Autodesk Inventor part; units mm, degrees
ref_plane "YZ Plane" through (0, 0, 0) normal (1, 0, 0) x (0, 1, 0)
ref_plane "XZ Plane" through (0, 0, 0) normal (0, 1, 0) x (-1, 0, 0)
ref_plane "XY Plane" through (0, 0, 0) normal (0, 0, 1) x (1, 0, 0)
sketch "Sketch4" plane through (0, 0, 0) normal (1, 0, 0) x (0, 1, 0)
  ellipse E0 centre (0, 0) end of major axis (-20, 0) minor radius 10
  dimension "d32" = 20
  dimension "d33" = 10
extrude "Extrusion1" add sketch "Sketch4" along normal blind 280
sketch "Sketch5" plane through (0, 0, 0) normal (-1, 0, 0) x (0, 0, 1)
  ellipse E0 centre (0, 0) end of major axis (0, 40) minor radius 40
  ellipse E1 centre (0, 0) end of major axis (0, -20) minor radius 10
  line L0 (0, 0) -> (0, 40)
  line L1 (0, 0) -> (-20, 34.641)
  line L2 (0, 0) -> (-34.641, 20)
  line L3 (0, 0) -> (-40, 0)
  line L4 (0, 0) -> (-34.641, -20)
  line L5 (0, 0) -> (-20, -34.641)
  line L6 (0, 0) -> (0, -40)
  line L7 (0, 0) -> (20, -34.641)
  line L8 (0, 0) -> (34.641, -20)
  line L9 (0, 0) -> (40, 0)
  line L10 (0, 0) -> (34.641, 20)
  line L11 (0, 0) -> (20, 34.641)
  line L12 (0, 23.094) -> (3.6979, 33.254)
  line L13 (2.2062, 35.3845) -> (0, 35.3845)
  arc A0 (3.6979, 33.254) -> (2.2062, 35.3845) centre (2.2062, 33.797) ccw
  line L14 (0, 23.094) -> (-3.6979, 33.254)
  line L15 (-2.2062, 35.3845) -> (0, 35.3845)
  arc A1 (-2.2062, 35.3845) -> (-3.6979, 33.254) centre (-2.2062, 33.797) ccw
  line L16 (-15.7816, 31.7469) -> (-17.6922, 30.6438)
  line L17 (-19.6028, 29.5408) -> (-17.6922, 30.6438)
  arc A2 (-19.6028, 29.5408) -> (-19.8295, 26.9498) centre (-18.8091, 28.1659) ccw
  line L18 (-11.547, 20) -> (-19.8295, 26.9498)
  line L19 (-11.547, 20) -> (-13.4245, 30.6478)
  arc A3 (-13.4245, 30.6478) -> (-15.7816, 31.7469) centre (-14.9879, 30.3721) ccw
  line L20 (-29.5408, 19.6028) -> (-30.6438, 17.6922)
  line L21 (-31.7469, 15.7816) -> (-30.6438, 17.6922)
  arc A4 (-31.7469, 15.7816) -> (-30.6478, 13.4245) centre (-30.3721, 14.9879) ccw
  line L22 (-20, 11.547) -> (-30.6478, 13.4245)
  line L23 (-20, 11.547) -> (-26.9498, 19.8295)
  arc A5 (-26.9498, 19.8295) -> (-29.5408, 19.6028) centre (-28.1659, 18.8091) ccw
  line L24 (-35.3845, 2.2062) -> (-35.3845, 0)
  line L25 (-35.3845, -2.2062) -> (-35.3845, 0)
  arc A6 (-35.3845, -2.2062) -> (-33.254, -3.6979) centre (-33.797, -2.2062) ccw
  line L26 (-23.094, 0) -> (-33.254, -3.6979)
  line L27 (-23.094, 0) -> (-33.254, 3.6979)
  arc A7 (-33.254, 3.6979) -> (-35.3845, 2.2062) centre (-33.797, 2.2062) ccw
  line L28 (-31.7469, -15.7816) -> (-30.6438, -17.6922)
  line L29 (-29.5408, -19.6028) -> (-30.6438, -17.6922)
  arc A8 (-29.5408, -19.6028) -> (-26.9498, -19.8295) centre (-28.1659, -18.8091) ccw
  line L30 (-20, -11.547) -> (-26.9498, -19.8295)
  line L31 (-20, -11.547) -> (-30.6478, -13.4245)
  arc A9 (-30.6478, -13.4245) -> (-31.7469, -15.7816) centre (-30.3721, -14.9879) ccw
  line L32 (-19.6028, -29.5408) -> (-17.6922, -30.6438)
  line L33 (-15.7816, -31.7469) -> (-17.6922, -30.6438)
  arc A10 (-15.7816, -31.7469) -> (-13.4245, -30.6478) centre (-14.9879, -30.3721) ccw
  line L34 (-11.547, -20) -> (-13.4245, -30.6478)
  line L35 (-11.547, -20) -> (-19.8295, -26.9498)
  arc A11 (-19.8295, -26.9498) -> (-19.6028, -29.5408) centre (-18.8091, -28.1659) ccw
  line L36 (-2.2062, -35.3845) -> (0, -35.3845)
  line L37 (2.2062, -35.3845) -> (0, -35.3845)
  arc A12 (2.2062, -35.3845) -> (3.6979, -33.254) centre (2.2062, -33.797) ccw
  line L38 (0, -23.094) -> (3.6979, -33.254)
  line L39 (0, -23.094) -> (-3.6979, -33.254)
  arc A13 (-3.6979, -33.254) -> (-2.2062, -35.3845) centre (-2.2062, -33.797) ccw
  line L40 (15.7816, -31.7469) -> (17.6922, -30.6438)
  line L41 (19.6028, -29.5408) -> (17.6922, -30.6438)
  arc A14 (19.6028, -29.5408) -> (19.8295, -26.9498) centre (18.8091, -28.1659) ccw
  line L42 (11.547, -20) -> (19.8295, -26.9498)
  line L43 (11.547, -20) -> (13.4245, -30.6478)
  arc A15 (13.4245, -30.6478) -> (15.7816, -31.7469) centre (14.9879, -30.3721) ccw
  line L44 (29.5408, -19.6028) -> (30.6438, -17.6922)
  line L45 (31.7469, -15.7816) -> (30.6438, -17.6922)
  arc A16 (31.7469, -15.7816) -> (30.6478, -13.4245) centre (30.3721, -14.9879) ccw
  line L46 (20, -11.547) -> (30.6478, -13.4245)
  line L47 (20, -11.547) -> (26.9498, -19.8295)
  arc A17 (26.9498, -19.8295) -> (29.5408, -19.6028) centre (28.1659, -18.8091) ccw
  line L48 (35.3845, -2.2062) -> (35.3845, 0)
  line L49 (35.3845, 2.2062) -> (35.3845, 0)
  arc A18 (35.3845, 2.2062) -> (33.254, 3.6979) centre (33.797, 2.2062) ccw
  line L50 (23.094, 0) -> (33.254, 3.6979)
  line L51 (23.094, 0) -> (33.254, -3.6979)
  arc A19 (33.254, -3.6979) -> (35.3845, -2.2062) centre (33.797, -2.2062) ccw
  line L52 (31.7469, 15.7816) -> (30.6438, 17.6922)
  line L53 (29.5408, 19.6028) -> (30.6438, 17.6922)
  arc A20 (29.5408, 19.6028) -> (26.9498, 19.8295) centre (28.1659, 18.8091) ccw
  line L54 (20, 11.547) -> (26.9498, 19.8295)
  line L55 (20, 11.547) -> (30.6478, 13.4245)
  arc A21 (30.6478, 13.4245) -> (31.7469, 15.7816) centre (30.3721, 14.9879) ccw
  line L56 (19.6028, 29.5408) -> (17.6922, 30.6438)
  line L57 (15.7816, 31.7469) -> (17.6922, 30.6438)
  arc A22 (15.7816, 31.7469) -> (13.4245, 30.6478) centre (14.9879, 30.3721) ccw
  line L58 (11.547, 20) -> (13.4245, 30.6478)
  line L59 (11.547, 20) -> (19.8295, 26.9498)
  arc A23 (19.8295, 26.9498) -> (19.6028, 29.5408) centre (18.8091, 28.1659) ccw
  line L60 (-3.175, 3.5066) -> (3.175, 3.5066)
  line L61 (3.175, 3.5066) -> (3.175, -3.5066)
  line L62 (3.175, -3.5066) -> (-3.175, -3.5066)
  line L63 (-3.175, -3.5066) -> (-3.175, 3.5066)
  line L64 (-3.175, 3.5066) -> (3.175, -3.5066) construction
  line L65 (3.175, 3.5066) -> (-3.175, -3.5066) construction
  dimension "d36" = 40
  dimension "d40" = 40
  dimension "d43" = 360
  dimension "d45" = 1.5875
  dimension "d46" = 10.16
  dimension "d47" = 20
  dimension "d50" = 360
  dimension "d52" = 6.35
extrude "Extrusion2" add sketch "Sketch5" against normal blind 1.25 contours L0 L15 A1 L14 E1 L1 L19 A3 L16 E0 | E0 L11 L57 A22 L58 E1 L0 L12 A0 L13 | L1 L17 A2 L18 E1 L2 L23 A5 L20 E0 | E0 L10 L53 A20 L54 E1 L11 L59 A23 L56 | L2 L21 A4 L22 E1 L3 L27 A7 L24 E0 | E0 L9 L49 A18 L50 E1 L10 L55 A21 L52 | L3 L25 A6 L26 E1 L4 L31 A9 L28 E0 | E0 L8 L45 A16 L46 E1 L9 L51 A19 L48 | L4 L29 A8 L30 E1 L5 L35 A11 L32 E0 | E0 L7 L41 A14 L42 E1 L8 L47 A17 L44 | L5 L33 A10 L34 E1 L6 L39 A13 L36 E0 | E0 L6 L37 A12 L38 E1 L7 L43 A15 L40
extrude "Extrusion3" cut sketch "Sketch5" against normal blind 6.35 contours L60 L11 L0 | L0 L1 L60 | L1 L2 L63 L60 | L60 L61 L10 L11 | L3 L63 L2 | L4 L63 L3 | L5 L62 L63 L4 | L6 L62 L5 | L7 L62 L6 | L8 L61 L62 L7 | L9 L61 L8 | L10 L61 L9
equation "\"d33\" = 0.5 * d32"
equation "\"d36\" = d40"
properties part number "tanjiro's sword hold"
The listing builds one solid part. Answer for the finished solid, in the listing's coordinates (mm). A direction names the side the tool comes from. Coordinates: 2 decimals unless noted, no trailing zeros. Put each result on its own line as item: value. Start each with the question number.
1. Flat-ended cylindrical pins translate along their axes: P1, Ø5, axis at y = -0.5, z = 0, coming from the -X side; P2, Ø3, axis at x = 4.5, z = 0, coming from the -Y side; P3, Ø2, axis at y = -13, z = -10.5, coming from the +X side. Find the tip coordinate at first contact, or state that the pin passes through.
2. For a pull along Y with two mould halves and no side action, classify faces 1 (the flat face through (280, 0, 0)), 2 (the flat face through (0.6, -23.4, -15.6)) as pulls with the +Y half, pulls with the -Y half, needs draft (parallel to the pull), parting line crosses it, or undercut.
3. Which of the six approach directions +Z, -Z, +X, -X, +Y, -Y give full straight-line access (tool end or side, diameter ignored) to faces 3 (the flat face through (3, -3.507, 0)), 4 (the flat face through (0, 1, 8)), 5 (the flat face through (1.25, -8.3, -9.4))?
4. Consider line 1 (X direction, y = 0, z = 16.5); line 2 (Z direction, x = 231, y = -18.5); line 3 (Z direction, x = 229, y = 1). Determine where each line is inside the solid, lowest interval first. Write a range as from..to.
Resolved:
1. P1: stops at x = 6.35
1. P2: stops at y = -20
1. P3: stops at x = 1.25
2. face 1: needs draft
2. face 2: undercut
3. face 3: -X
3. face 4: +Z, -Z, -X, +Y, -Y
3. face 5: +X
4. line 1: x = 0..1.25
4. line 2: z = -3.8..3.8
4. line 3: z = -9.99..9.99
